Could you check a few things on this model? Use its own coordinates, in mm. A direction names the side the tool comes from. Coordinates: 2 decimals unless noted, no trailing zeros. Write each loop counter-clockwise with the first axis right and the second up, starting at its lowest first coordinate (ties: lowest second). Pieces come first, ordered by that corner, then holes. Notation, with made-up numbers: (80, -13.5) - (115, -13.5) arc R4 cw to (115, -8.5) - close; hole circle Ø1 at (-14.5, -36.5). An arc over 180 degrees is marked (long way). Answer as a JSON object with one key per item and string values. Group by question number.
1) Will these pins go through, and if not, where does the flat tip stop? pin 1 Ø8 at (x, y) = (-25.5, 9) entering from +Z; pin 2 Ø10 at (x, y) = (-50, 21) entering from -Z; pin 3 Ø3 at (y, z) = (1.5, 46.5) entering from +X.
2) Please list where these lines run through material, in increasing order: line 1 along X through (y, z) = (10.25, 0); line 2 along Y through (x, z) = (67, 24); line 3 along Z through (x, y) = (7, 7.75).
3) If we section it at C-C (z = 38.5): Write out the boundary of the cut face in (x, y), plus the area to 3 significant figures.
4) If we section it at B-B (z = -52): Write out the boundary of the cut face in (x, y), plus the area to 3 significant figures.
5) On a 3-axis mill with a long thin cutter (end or side, diameter ignored), from which of +Z, -Z, +X, -X, +Y, -Y can I reach the whole of each face in a straight line? I mean faces 4 (the cylindrical face through (9.58, 1.25, 13.29)), 5 (the flat face through (0, 2.54, -1)). Say none if no direction works.
6) If we section it at D-D (y = 7): Write out the boundary of the cut face in (x, z).
7) We'd pull the mould along X, two halves only. Please class faces 1 (the flat face through (-76, 25.4, 17)), 2 (the cylindrical face through (-9.68, 1.25, 13.22)), 3 (the cylindrical face through (23.865, 12.522, 75.782)): released by +X, released by -X, zero draft, split by the parting line, or undercut.
8) If we section it at A-A (x = 0): Write out the boundary of the cut face in (y, z).
```python
from build123d import *

# Parameters (mm, degrees)
SKETCH1_R           = 16.383937572
BOSS_EXTRUDE1_DEPTH = 2.54
SKETCH2_R           = 79.4512
SKETCH2_R_2         = 77.47
BOSS_EXTRUDE2_DEPTH = 25.4
FILLET2_R           = 7.62
FILLET3_R           = 5.08


with BuildPart() as part:
    # Sketch1 → Boss-Extrude1 (new body)
    with BuildSketch(Plane(origin=(0, 0, 0), x_dir=(1, 0, 0), z_dir=(0, 1, 0))):
        Circle(SKETCH1_R)
        with BuildLine():
            ThreePointArc((-11.540007509, 11.630203655), (-9.630236879, 13.254883931), (-7.494922537, 14.569129917))
            Line((-7.494922537, 14.569129917), (-43.513181009, 64.144009685))
            Line((-43.513181009, 64.144009685), (-47.558265981, 61.205083423))
            Line((-47.558265981, 61.205083423), (-11.540007509, 11.630203655))
        make_face()
        with BuildLine():
            Line((43.513181009, 64.144009685), (7.494922537, 14.569129917))
            ThreePointArc((7.494922537, 14.569129917), (9.630236879, 13.254883931), (11.540007509, 11.630203655))
            Line((11.540007509, 11.630203655), (47.558265981, 61.205083423))
            Line((47.558265981, 61.205083423), (43.513181009, 64.144009685))
        make_face()
        with BuildLine():
            Line((74.450890803, -21.561905263), (16.17212438, -2.62598618))
            ThreePointArc((16.17212438, -2.62598618), (15.582050591, -5.062915145), (14.627039408, -7.381268762))
            Line((14.627039408, -7.381268762), (72.905805831, -26.317187845))
            Line((72.905805831, -26.317187845), (74.450890803, -21.561905263))
        make_face()
        with BuildLine():
            Line((2.5, -77.47), (2.5, -16.19207863))
            ThreePointArc((2.5, -16.19207863), (0, -16.383937572), (-2.5, -16.19207863))
            Line((-2.5, -16.19207863), (-2.5, -77.47))
            Line((-2.5, -77.47), (2.5, -77.47))
        make_face()
        with BuildLine():
            ThreePointArc((-14.627039408, -7.381268762), (-15.582050591, -5.062915145), (-16.17212438, -2.62598618))
            Line((-16.17212438, -2.62598618), (-74.450890803, -21.561905263))
            Line((-74.450890803, -21.561905263), (-72.905805831, -26.317187845))
            Line((-72.905805831, -26.317187845), (-14.627039408, -7.381268762))
        make_face()
    extrude(amount=BOSS_EXTRUDE1_DEPTH)

    # Sketch2 → Boss-Extrude2 (add)
    with BuildSketch(Plane(origin=(0, 0, 0), x_dir=(1, 0, 0), z_dir=(0, 1, 0))):
        with Locations(Location((0, 0, 0), (0, 0, 270))):
            Circle(SKETCH2_R)
        with Locations(Location((0, 0, 0), (0, 0, 124.150712253))):
            Circle(SKETCH2_R_2, mode=Mode.SUBTRACT)
    extrude(amount=BOSS_EXTRUDE2_DEPTH)

    # Fillet2
    fillet2_edges = [part.edges().sort_by_distance(p)[0] for p in [
        (72.867431935, 1.27, 26.30471941),
        (47.534549609, 1.27, -61.172440637),
        (-43.489464637, 1.27, -64.111366899),
        (-74.412516907, 1.27, 21.549436829),
        (-2.5, 1.27, 77.429651297),
        (-47.534549609, 1.27, -61.172440637),
        (43.489464637, 1.27, -64.111366899),
        (74.412516907, 1.27, 21.549436829),
        (2.5, 1.27, 77.429651297),
        (-72.867431935, 1.27, 26.30471941),
    ]]
    fillet(fillet2_edges, radius=FILLET2_R)

    # Fillet3
    fillet3_edges = [part.edges().sort_by_distance(p)[0] for p in [
        (-2.5, 1.27, 16.19207863),
        (-14.627039408, 1.27, 7.381268762),
        (-16.17212438, 1.27, 2.62598618),
        (-11.540007509, 1.27, -11.630203655),
        (-7.494922537, 1.27, -14.569129917),
        (7.494922537, 1.27, -14.569129917),
        (11.540007509, 1.27, -11.630203655),
        (16.17212438, 1.27, 2.62598618),
        (14.627039408, 1.27, 7.381268762),
        (2.5, 1.27, 16.19207863),
    ]]
    fillet(fillet3_edges, radius=FILLET3_R)


solid = part.part
```
Here are the results:
{
 "1": {"pin 1": "stops at z = 76.49", "pin 2": "stops at z = -65.48", "pin 3": "stops at x = 65.48"},
 "2": {"line 1": "x = -79.45 to -77.47, 77.47 to 79.45", "line 2": "y = 0 to 2.54", "line 3": "z = -79.14 to -77.15, 77.15 to 79.14"},
 "3": {"outline": "(-69.5, 0) - (-67.23, 0) - (-67.23, 25.4) - (-69.5, 25.4) - close; (-2.5, 0) - (2.5, 0) - (2.5, 2.54) - (-2.5, 2.54) - close; (67.23, 0) - (69.5, 0) - (69.5, 25.4) - (67.23, 25.4) - close", "area": "128 mm²"},
 "4": {"outline": "(-60.07, 0) - (-57.42, 0) - (-57.42, 25.4) - (-60.07, 25.4) - close; (-40.87, 0) - (-34.69, 0) - (-34.69, 2.54) - (-40.87, 2.54) - close; (34.69, 0) - (40.87, 0) - (40.87, 2.54) - (34.69, 2.54) - close; (57.42, 0) - (60.07, 0) - (60.07, 25.4) - (57.42, 25.4) - close", "area": "166 mm²"},
 "5": {"face 4": "+Y, -Y", "face 5": "+Y"},
 "6": {"outline": "circle Ø158.9 at (0, 0); hole circle Ø154.94 at (0, 0)"},
 "7": {"face 1": "zero draft", "face 2": "undercut", "face 3": "split by the parting line"},
 "8": {"outline": "(0, -79.45) - (25.4, -79.45) - (25.4, -77.47) - (0, -77.47) - close; (0, -16.38) - (2.54, -16.38) - (2.54, 77.47) - (25.4, 77.47) - (25.4, 79.45) - (0, 79.45) - close"}
}
